```python
from build123d import *

# Parameters (mm, degrees)
P_IDAT_VYSUNUT_M2_DEPTH  = 10
SKICA2_R                 = 21
P_IDAT_VYSUNUT_M3_DEPTH  = 22
SKICA3_R                 = 12.8
SKICA3_W                 = 7
SKICA3_H                 = 3.487810918
ODEBRAT_VYSUNUT_M1_DEPTH = 61
ZKOSEN_3_SIZE            = 0.5


with BuildPart() as part:
    # Skica1 → Přidat vysunutím2 (new body)
    with BuildSketch(Plane.XY):
        with BuildLine():
            ThreePointArc((38.9875, -8.942865522), (31, 0), (38.9875, 8.942865522))
            ThreePointArc((38.9875, 8.942865522), (38.637033052, 10.352761804), (38.235598191, 11.749001275))
            ThreePointArc((38.235598191, 11.749001275), (26.846787517, 15.5), (29.292732669, 27.238498725))
            ThreePointArc((29.292732669, 27.238498725), (28.284271247, 28.284271247), (27.238498725, 29.292732669))
            ThreePointArc((27.238498725, 29.292732669), (15.5, 26.846787517), (11.749001275, 38.235598191))
            ThreePointArc((11.749001275, 38.235598191), (10.352761804, 38.637033052), (8.942865522, 38.9875))
            ThreePointArc((8.942865522, 38.9875), (0, 31), (-8.942865522, 38.9875))
            ThreePointArc((-8.942865522, 38.9875), (-10.352761804, 38.637033052), (-11.749001275, 38.235598191))
            ThreePointArc((-11.749001275, 38.235598191), (-15.5, 26.846787517), (-27.238498725, 29.292732669))
            ThreePointArc((-27.238498725, 29.292732669), (-28.284271247, 28.284271247), (-29.292732669, 27.238498725))
            ThreePointArc((-29.292732669, 27.238498725), (-26.846787517, 15.5), (-38.235598191, 11.749001275))
            ThreePointArc((-38.235598191, 11.749001275), (-38.637033052, 10.352761804), (-38.9875, 8.942865522))
            ThreePointArc((-38.9875, 8.942865522), (-31, 0), (-38.9875, -8.942865522))
            ThreePointArc((-38.9875, -8.942865522), (-38.637033052, -10.352761804), (-38.235598191, -11.749001275))
            ThreePointArc((-38.235598191, -11.749001275), (-26.846787517, -15.5), (-29.292732669, -27.238498725))
            ThreePointArc((-29.292732669, -27.238498725), (-28.284271247, -28.284271247), (-27.238498725, -29.292732669))
            ThreePointArc((-27.238498725, -29.292732669), (-15.5, -26.846787517), (-11.749001275, -38.235598191))
            ThreePointArc((-11.749001275, -38.235598191), (-10.352761804, -38.637033052), (-8.942865522, -38.9875))
            ThreePointArc((-8.942865522, -38.9875), (0, -31), (8.942865522, -38.9875))
            ThreePointArc((8.942865522, -38.9875), (10.352761804, -38.637033052), (11.749001275, -38.235598191))
            ThreePointArc((11.749001275, -38.235598191), (15.5, -26.846787517), (27.238498725, -29.292732669))
            ThreePointArc((27.238498725, -29.292732669), (28.284271247, -28.284271247), (29.292732669, -27.238498725))
            ThreePointArc((29.292732669, -27.238498725), (26.846787517, -15.5), (38.235598191, -11.749001275))
            ThreePointArc((38.235598191, -11.749001275), (38.637033052, -10.352761804), (38.9875, -8.942865522))
        make_face()
        with BuildLine():
            Line((-3.5, 12.312189082), (-3.5, 15.8))
            Line((-3.5, 15.8), (3.5, 15.8))
            Line((3.5, 15.8), (3.5, 12.312189082))
            ThreePointArc((3.5, 12.312189082), (0, -12.8), (-3.5, 12.312189082))
        make_face(mode=Mode.SUBTRACT)
    extrude(amount=P_IDAT_VYSUNUT_M2_DEPTH)

    # Skica2 → Přidat vysunutím3 (add)
    with BuildSketch(Plane.XY.offset(10)):
        Circle(SKICA2_R)
    extrude(amount=P_IDAT_VYSUNUT_M3_DEPTH)

    # Skica3 → Odebrat vysunutím1 (cut)
    with BuildSketch(Plane(origin=(0, 0, 0), x_dir=(-1, 0, 0), z_dir=(0, 0, -1))):
        Circle(SKICA3_R)
        with Locations((0, 14.056094541)):
            Rectangle(SKICA3_W, SKICA3_H)
    extrude(amount=-ODEBRAT_VYSUNUT_M1_DEPTH, mode=Mode.SUBTRACT)

    # Zkosení3
    zkosen_3_edges = [part.edges().sort_by_distance(p)[0] for p in [
        (-21, 0, 32),
    ]]
    chamfer(zkosen_3_edges, length=ZKOSEN_3_SIZE)


solid = part.part
```
Work out the finished part from the listing and answer in its coordinate system (mm). A direction names the side the tool comes from. Give positions to 0.01 mm unless a question says otherwise; leave off trailing zeros. Loops run counter-clockwise (first coordinate to the right, second up) from the corner with the lowest first, then second, coordinate; pieces in that order, holes last. Notation, with made-up numbers: (84, -21) -> (92, -21) arc R17 cw to (92, -3) -> close; hole circle Ø10 at (-39, 16). An arc over 180 degrees is marked (long way). Use CSV: the item, a comma, the result in double quotes.
1. A tool of negligible diameter and unlimited length cuts with its end or side. For faces 5 (the flat face through (0, 15.8, 16)), 6 (the flat face through (0, -13, 32)), 7 (the cylindrical face through (20.03, 6.31, 20.6)), from which of +Z, -Z, +X, -X, +Y, -Y can it reach the whole face along a straight path? Write none if from no direction.
Found:
face 5,"+Z, -Z"
face 6,"+Z, +X, -X, +Y, -Y"
face 7,"+Z"
2. The part is cut by section A-A (y = 0). Write down the section's boundary in (x, z), then the cut area to 3 significant figures.
Found:
outline,"(-31, 0) -> (-12.8, 0) -> (-12.8, 32) -> (-20.5, 32) -> (-21, 31.5) -> (-21, 10) -> (-31, 10) -> close; (12.8, 0) -> (31, 0) -> (31, 10) -> (21, 10) -> (21, 31.5) -> (20.5, 32) -> (12.8, 32) -> close"
area,"725 mm^2"
3. The part is cut by section C-C (z = 19.5). Write down the section's boundary in (x, y), then the cut area to 3 significant figures.
Found:
outline,"circle Ø42 at (0, 0); hole (-3.5, 12.31) arc R12.8 ccw (long way) to (3.5, 12.31) -> (3.5, 15.8) -> (-3.5, 15.8) -> close"
area,"849 mm^2"
4. The mould has two halves that part along X. Classify faces 1 (the cylindrical face through (26.94, 15.34, 4.93)), 2 (the cylindrical face through (38.632, -10.372, 4.93)), 3 (the flat face through (17, -17, 10)), 4 (the cylindrical face through (-10.333, 38.642, 4.93)): +X half, -X half, draft (parallel to the pull), parting line (faces both ways), or undercut.
Found:
face 1,"undercut"
face 2,"+X half"
face 3,"draft"
face 4,"-X half"
5. Straight lines are drawn through the part: line 1 (Y direction, x = 0, z = 13); line 2 (Y direction, x = -0.5, z = 6.5); line 3 (Y direction, x = 27, z = 6). For each, find the intervals that lie inside material, in ascending order.
Found:
line 1,"-21 to -12.8, 15.8 to 21"
line 2,"-31.01 to -12.79, 15.8 to 31.01"
line 3,"-28.98 to -24.76, -15.24 to 15.24, 24.76 to 28.98"
6. The part is cut by section B-B (x = 0). Write down the section's boundary in (y, z), then the cut area to 3 significant figures.
Found:
outline,"(-31, 0) -> (-12.8, 0) -> (-12.8, 32) -> (-20.5, 32) -> (-21, 31.5) -> (-21, 10) -> (-31, 10) -> close; (15.8, 0) -> (31, 0) -> (31, 10) -> (21, 10) -> (21, 31.5) -> (20.5, 32) -> (15.8, 32) -> close"
area,"629 mm^2"
7. Flat-ended cylindrical pins translate along their axes: pin 1 Ø15.5 at (x, y) = (0, 0) entering from +Z; pin 2 Ø3 at (y, z) = (10.5, 21.5) entering from +X; pin 3 Ø5 at (x, z) = (-19, 12) entering from +Y; pin 4 Ø8 at (y, z) = (-4, 7.5) entering from +X. Find the tip coordinate at first contact, or state that the pin passes through.
Found:
pin 1,"through"
pin 2,"x = 18.97"
pin 3,"y = 26"
pin 4,"x = 35.88"
8. The part is cut by section D-D (x = 32). Write down the section's boundary in (y, z), then the cut area to 3 significant figures.
Found:
outline,"(-11.4, 0) -> (-4.12, 0) -> (-4.12, 10) -> (-11.4, 10) -> close; (4.12, 0) -> (11.4, 0) -> (11.4, 10) -> (4.12, 10) -> close"
area,"145 mm^2"
